Can you work these out from the model? Positions are in its coordinate system, mm. A direction names the side the tool comes from. Coordinates: 2 decimals unless noted, no trailing zeros. Write each loop counter-clockwise with the first axis right and the second up, starting at its lowest first coordinate (ties: lowest second). Pieces come first, ordered by that corner, then holes. Notation, with made-up numbers: (31.25, 45) - (59.25, 45) arc R22 ccw to (59.25, 65) - close; hole circle Ø1 at (46.5, 26). An arc over 180 degrees is marked (long way). Use one line per item in the form item = value. Start each with the question number.
(1) If we section it at B-B on x = 0: Please give me the cut outline in (y, z) (3 decimals).
(2) Thinking about a two-plate mould opening in Z: for faces 1 (the face through (-9.05, 19.64, 17.4)), 2 (the face through (12.2, -29.35, -4.2)), 3 (the face through (11.012, -0.184, 49.592)), which applies, pulls with the +Z half, pulls with the -Z half, needs draft (parallel to the pull), parting line crosses it, or undercut?
(3) If we section it at C-C on y = 13.5: Please give me the cut outline in (x, z) (3 decimals).
(4) For pin 1 Ø20.5 at (x, z) = (17.46, 30.25) entering from +Y; pin 2 Ø5 at (x, y) = (-36, -16) entering from -Z; pin 3 Ø5 at (y, z) = (-5.5, 5.5) entering from -X, each with a flat end and sliding along its axis, tell me the tip position at first contact or that it passes through.
(5) On a 3-axis mill with a long thin cutter (end or side, diameter ignored), from which of +Z, -Z, +X, -X, +Y, -Y can I reach the whole of each face in a straight line? I mean faces 4 (the face through (-40.98, -0.07, -1.91)), 5 (the face through (20.5, 4.826, 9.9)), 6 (the face through (15.3, -22.098, -45.4)). Say none if no direction works.
(6) If we section it at D-D on x = 32: Please give me the cut outline in (y, z), then the cut area to 3 significant figures.
(7) If I drill on probe 1 along X at (y, z) = (10, 0) (3 decimals); probe 2 along Z at (x, y) = (8, -8); probe 3 along X at (y, z) = (10.5, -16), over which ranges is the centre line in solid material (lowest first)? Write a range as from..to.
(8) If we section it at A-A on z = 0: Give the number of separate pieces and of enclosed holes in the cut face, then the cut area to 3 significant figures.
```python
from build123d import *

# Parameters (mm, degrees)
F_1_2_0_5_DIAMETER_HOLE1_D = 12.7


with BuildPart() as part:
    # Sketch1 → Revolve1 (revolve)
    with BuildSketch(Plane.XY):
        Polygon((-12.7, 29.3497), (-17.900810023, 29.3497), (-22.225, 4.826), (-47.625, 4.826), (-47.625, 22.352), (-50.8, 22.352), (-50.8, -22.098), (-47.625, -22.098), (-47.625, -4.826), (-22.225, -4.826), (-17.900810023, -29.3497), (-12.7, -29.3497), align=None)
    revolve(axis=Axis((0, 29.3497, 0), (0, -1, 0)))

    # 1/2 (0.5) Diameter Hole1 (through all)
    with Locations(Plane(origin=(0, 4.826, 0), x_dir=(1, 0, 0), z_dir=(0, 1, 0))):
        with Locations((-17.4625, 30.245937227), (17.4625, 30.245937227), (-34.925, 0), (34.925, 0), (-17.4625, -30.245937227), (17.4625, -30.245937227)):
            Hole(F_1_2_0_5_DIAMETER_HOLE1_D / 2)


solid = part.part
```
Reported:
q1.outline = (-29.35, -17.901) - (-4.826, -22.225) - (-4.826, -47.625) - (-22.098, -47.625) - (-22.098, -50.8) - (22.352, -50.8) - (22.352, -47.625) - (4.826, -47.625) - (4.826, -22.225) - (29.35, -17.901) - (29.35, -12.7) - (-29.35, -12.7) - close; (-29.35, 12.7) - (29.35, 12.7) - (29.35, 17.901) - (4.826, 22.225) - (4.826, 47.625) - (22.352, 47.625) - (22.352, 50.8) - (-22.098, 50.8) - (-22.098, 47.625) - (-4.826, 47.625) - (-4.826, 22.225) - (-29.35, 17.901) - close
q2.face_1 = undercut
q2.face_2 = needs draft
q2.face_3 = parting line crosses it
q3.outline = circle Ø101.6 at (0, 0); circle Ø41.391 at (0, 0); hole circle Ø95.25 at (0, 0); hole circle Ø25.4 at (0, 0)
q4.pin_1 = 4.83
q4.pin_2 = -38.19
q4.pin_3 = -50.71
q5.face_4 = +Y, -Y
q5.face_5 = +Y
q5.face_6 = -Y
q6.outline = (-22.1, -39.45) - (22.35, -39.45) - (22.35, -35.27) - (4.83, -35.27) - (4.83, -5.64) - (-4.83, -5.64) - (-4.83, -35.27) - (-22.1, -35.27) - close; (-22.1, 35.27) - (-4.83, 35.27) - (-4.83, 5.64) - (4.83, 5.64) - (4.83, 35.27) - (22.35, 35.27) - (22.35, 39.45) - (-22.1, 39.45) - close
q6.area = 944 mm2
q7.probe_1 = -50.8..-47.625, -21.313..-12.7, 12.7..21.313, 47.625..50.8
q7.probe_2 = -50.17..-46.95, -20.13..-9.86, 9.86..20.13, 46.95..50.17
q7.probe_3 = -48.21..-44.86, -13.95..13.95, 44.86..48.21
q8.separate_pieces = 4
q8.enclosed_holes = 0
q8.area = 1,430 mm2
